Check sheet for the modelled part. Datum: model origin and axes. Units: mm. A direction names the side the tool comes from. Give positions to 0.01 mm unless a question says otherwise; leave off trailing zeros. Loops run counter-clockwise (first coordinate to the right, second up) from the corner with the lowest first, then second, coordinate; pieces in that order, holes last.
```python
from build123d import *

# Parameters (mm, degrees)
BOSS_EXTRUDE1_DEPTH = 6


with BuildPart() as part:
    # Sketch1 → Boss-Extrude1 (new body)
    with BuildSketch(Plane(origin=(0, 0, 0), x_dir=(1, 0, 0), z_dir=(0, 1, 0))):
        with BuildLine():
            Line((-0.334505703, -6.891886965), (262.047385932, -19.626895486))
            ThreePointArc((262.047385932, -19.626895486), (282.65, 0), (262.047385932, 19.626895486))
            Line((262.047385932, 19.626895486), (-0.334505703, 6.891886965))
            ThreePointArc((-0.334505703, 6.891886965), (-6.9, 0), (-0.334505703, -6.891886965))
        make_face()
        with BuildLine():
            Line((-0.295722433, 6.092827606), (262.086169202, 18.827836128))
            ThreePointArc((262.086169202, 18.827836128), (281.85, 0), (262.086169202, -18.827836128))
            Line((262.086169202, -18.827836128), (-0.295722433, -6.092827606))
            ThreePointArc((-0.295722433, -6.092827606), (-6.1, 0), (-0.295722433, 6.092827606))
        make_face(mode=Mode.SUBTRACT)
    extrude(amount=BOSS_EXTRUDE1_DEPTH)


solid = part.part
```
(1) Gauge pin test, flat ends, axial feed: pin 1 Ø2 at (y, z) = (1.5, -12) entering from +X; pin 2 Ø1 at (x, y) = (132, 1.5) entering from +Z; pin 3 Ø8 at (x, z) = (130, 6) entering from -Y; pin 4 Ø3 at (x, y) = (76.5, 2) entering from -Z. Record the tip position at first contact, or that the pin passes through.
(2) Section check B-B on y = 4.2. Record the boundary of the cut face in (x, z), plus the area to 3 significant figures.
(3) Section check A-A on z = 0. Record the boundary of the cut face in (x, y), plus the area to 3 significant figures.
(4) Section check C-C on x = 183.5. Record the boundary of the cut face in (y, z), plus the area to 3 significant figures.
(5) Access from +Z, -Z, +X, -X, +Y, -Y to the whole of each face (thin tool, end or side, straight path). Record for faces 4 (the face through (281.845, 2.958, -0.427)), 5 (the face through (137, 0, -13)).
(6) Release check for a two-part mould opening along Z. For faces 1 (the face through (137, 6, -13)), 2 (the face through (-6.9, 3, -0.1)), 3 (the face through (132.73, 2.96, 12.55)) record: pulls with the +Z half, pulls with the -Z half, needs draft (parallel to the pull), parting line crosses it, or undercut.
(7) Material ranges on line 1 (Z direction, x = 263.5, y = 0.25); line 2 (X direction, y = 2.45, z = -0.5); line 3 (X direction, y = 2.1, z = 3), recorded low to high.
Computed values:
1. pin 1: stops at x = 279.28
1. pin 2: stops at z = 13.34
1. pin 3: passes through
1. pin 4: stops at z = -10.69
2. outline: (-0.33, -6.89) - (262.05, -19.63) arc R19.65 ccw (long way) to (262.05, 19.63) - (-0.33, 6.89) arc R6.9 ccw to start; hole (-0.3, -6.09) - (262.09, -18.83) arc R18.85 ccw (long way) to (262.09, 18.83) - (-0.3, 6.09) arc R6.1 ccw to start
2. area: 486 mm2
3. outline: (-6.9, 0) - (-6.1, 0) - (-6.1, 6) - (-6.9, 6) - close; (281.85, 0) - (282.65, 0) - (282.65, 6) - (281.85, 6) - close
3. area: 9.60 mm2
4. outline: (0, -15.81) - (6, -15.81) - (6, -15.01) - (0, -15.01) - close; (0, 15.01) - (6, 15.01) - (6, 15.81) - (0, 15.81) - close
4. area: 9.61 mm2
5. face 4: +Y, -Y
5. face 5: +Z, -Z, +X, -X, -Y
6. face 1: needs draft
6. face 2: parting line crosses it
6. face 3: undercut
7. line 1: z = -19.64 to -18.84, 18.84 to 19.64
7. line 2: x = -6.88 to -6.08, 281.84 to 282.64
7. line 3: x = -6.21 to -5.31, 281.61 to 282.42
